Verification items for the finished model (mm, model axes). Coordinates: 2 decimals unless noted, no trailing zeros. Loops run counter-clockwise (first coordinate to the right, second up) from the corner with the lowest first, then second, coordinate; pieces in that order, holes last.
Q1. Sectioned sample at A-A (x = 0). Enter the section's corners in (y, z).
Q2. Go/stop test with flat-tipped pins: P1, Ø5, axis at x = -3.5, y = 227, coming from the -Z side; P2, Ø6, axis at y = 104.5, z = 4.5, coming from the +X side; P3, Ø5, axis at x = -4.5, y = 233, coming from the -Z side. Record where each tip stops, or that it passes through.
Q3. Sectioned sample at C-C (y = 98.5). Enter the section's corners in (x, z).
Q4. Sectioned sample at D-D (y = 10). Enter the section's corners in (x, z), then the cut area to 3 significant figures.
Q5. Mould release check, pull along Z, two halves, no side actions. Record for faces 1 (the face through (4, 0, 4)), 2 (the face through (6, 148, 0)), 3 (the face through (4.99, 7.97, 2.21)): +Z half, -Z half, draft (parallel to the pull), parting line (faces both ways), or undercut.
Q6. Material ranges on probe 1 along Z at (x, y) = (0, 218); probe 2 along X at (y, z) = (270.5, 0.75), recorded low to high.
Q7. Sectioned sample at B-B (z = 0). Enter the section's corners in (x, y).
Autodesk Inventor part; units mm, degrees
ref_plane "Work Plane3" through (6, 0, 0) normal (1, 0, 0) x (0, 1, 0)
ref_plane "XZ Plane" through (0, 0, 0) normal (0, 1, 0) x (-1, 0, 0)
ref_plane "XY Plane" through (0, 0, 0) normal (0, 0, 1) x (1, 0, 0)
sketch "Sketch1" plane through (0, 0, 0) normal (0, 1, 0) x (-1, 0, 0)
  circle A0 centre (0, 0) radius 5
  circle A1 centre (0, 0) radius 6
  dimension "d0" = 12
  dimension "d1" = 1
extrude "Extrusion1" add sketch "Sketch1" along normal blind 300
ref_plane "Work Plane3" through (6, 0, 0) normal (1, 0, 0) x (0, 1, 0)
sketch "Sketch2" plane through (6, 0, 0) normal (1, 0, 0) x (0, 1, 0)
  line L0 (0, -6) -> (300, -6)
  line L1 (0, 6) -> (300, 6)
  line L2 (300, -6) -> (300, 6)
  line L3 (-60, 0) -> (360, 0)
  point P0 (0, 0)
  point P1 (10, 0)
  point P2 (292, 0)
  point P3 (300, 0)
  dimension "d20" = 10
  dimension "d21" = 8
hole "Hole1" at (6, 10, 0) direction (-1, 0, 0) diameter 6 end up to surface
hole "Hole2" at (6, 292, 0) direction (-1, 0, 0) diameter 4 end up to surface
equation "\"d2\" = pipe_length"
equation "\"pipe_length\" = 300"
properties part number "pipe" material "Aluminum 6061"
Geometry check:
1. outline: (0, -6) - (300, -6) - (300, -5) - (0, -5) - close; (0, 5) - (300, 5) - (300, 6) - (0, 6) - close
2. P1: stops at z = -5.92
2. P2: stops at x = 5.81
2. P3: stops at z = -5.66
3. outline: circle Ø12 at (0, 0); hole circle Ø10 at (0, 0)
4. outline: (4, -3) arc R5 cw (long way) to (4, 3) - (5.2, 3) arc R6 ccw (long way) to (5.2, -3) - close
4. area: 28.2 mm2
5. face 1: draft
5. face 2: parting line
5. face 3: undercut
6. probe 1: z = -6 to -5, 5 to 6
6. probe 2: x = -5.95 to -4.94, 4.94 to 5.95
7. outline: (-6, 0) - (-5, 0) - (-5, 300) - (-6, 300) - close; (5, 0) - (6, 0) - (6, 7) - (5, 7) - close; (5, 13) - (6, 13) - (6, 290) - (5, 290) - close; (5, 294) - (6, 294) - (6, 300) - (5, 300) - close
